from build123d import *

# Parameters (mm, degrees)
BOSS_EXTRUDE1_DEPTH     = 12.5
SKETCH2_W               = 12.5
SKETCH2_H               = 1.5
BOSS_EXTRUDE2_DEPTH     = 6
SKETCH3_R               = 1.5
CUT_EXTRUDE1_DEPTH      = 34.000006013
CUT_EXTRUDE1_DEPTH_BACK = 13.999994598
SKETCH5_W               = 1
SKETCH5_H               = 5
CUT_EXTRUDE2_DEPTH      = 24.499994598


with BuildPart() as part:
    # Sketch1 → Boss-Extrude1 (new body)
    with BuildSketch(Plane.XY):
        with BuildLine():
            Line((5.5, 17), (5.5, -18))
            ThreePointArc((5.5, -18), (-2.701e-06, -23.499994598), (-5.5, -17.999994598))
            Line((-5.5, -17.999994598), (-5.5, 17.000006013))
            ThreePointArc((-5.5, 17.000006013), (3.006e-06, 22.500006013), (5.5, 17))
        make_face()
        with BuildLine():
            Line((2.5, 17.5), (2.5, -17.5))
            ThreePointArc((2.5, -17.5), (0, -20), (-2.5, -17.5))
            Line((-2.5, -17.5), (-2.5, 17.5))
            ThreePointArc((-2.5, 17.5), (0, 20), (2.5, 17.5))
        make_face(mode=Mode.SUBTRACT)
    extrude(amount=BOSS_EXTRUDE1_DEPTH)

    # Sketch2 → Boss-Extrude2 (add)
    with BuildSketch(Plane(origin=(5.5, 0, 0), x_dir=(0, 0, -1), z_dir=(1, 0, 0))):
        with Locations((-6.25, -11.25)):
            Rectangle(SKETCH2_W, SKETCH2_H)
        with Locations((-6.25, -6.75)):
            Rectangle(SKETCH2_W, SKETCH2_H)
    extrude(amount=BOSS_EXTRUDE2_DEPTH)

    # Sketch3 → Cut-Extrude1 (cut, two sides)
    with BuildSketch(Plane(origin=(0, -10.5, 0), x_dir=(1, 0, 0), z_dir=(0, 1, 0))) as cut_extrude1_sk:
        with Locations((8.5, -3)):
            Circle(SKETCH3_R)
        with Locations((8.5, -9.5)):
            Circle(SKETCH3_R)
    extrude(amount=CUT_EXTRUDE1_DEPTH, mode=Mode.SUBTRACT)
    extrude(cut_extrude1_sk.sketch, amount=-CUT_EXTRUDE1_DEPTH_BACK, mode=Mode.SUBTRACT)

    # Sketch5 → Cut-Extrude2 (cut, through all)
    with BuildSketch(Plane(origin=(0, 0, 0), x_dir=(1, 0, 0), z_dir=(0, 1, 0))):
        with Locations((0, -6.25)):
            Rectangle(SKETCH5_W, SKETCH5_H)
    extrude(amount=-CUT_EXTRUDE2_DEPTH, mode=Mode.SUBTRACT)


solid = part.part
Here's how the part is built. I have some questions about the finished solid (model axes, mm). A direction names the side the tool comes from. Round coordinates to 2 decimals unless told otherwise and drop trailing zeros. Order: outer loops, then holes, each group sorted by start corner. A loop starts at its lowest first (then second) coordinate and runs counter-clockwise, first axis right, second up. Notation, with made-up numbers: M -24.75,-17.5 L -11.75,-17.5 A18 ccw -11.75,-8.5 Z; hole C 38,-19.5 d2. An arc over 180 degrees is marked long. Return JSON: item names as keys, results as strings. Group by question number.
1. If we section it at B-B on y = 2.5: List the corners of the cut face in (x, z) for me.
2. I'm going to push flat-ended pins straight in: pin 1 Ø5 at (y, z) = (-16, 8.5) entering from +X; pin 2 Ø2 at (x, y) = (4, 12.5) entering from -Z; pin 3 Ø1.1 at (y, z) = (-21, 5) entering from +X; pin 4 Ø3 at (x, z) = (8.5, 5.5) entering from -Y. Where does each tip first touch, or does it pass through?
3. If we mould it in two halves opening along X, with no side actions, what happens to faces 1 (the face through (1.994, -23.126, 6.162)), 2 (the face through (0, -22, 3.75)), 3 (the face through (-3, 0, 0))? For each: pulls with the +X half, pulls with the -X half, needs draft (parallel to the pull), parting line crosses it, or undercut.
4. If we section it at A-A on z = 9.5: List the corners of the cut face in (x, y) for me.
5. Please list where these lines run through material, in increasing order: probe 1 along X at (y, z) = (-10.95, 9.5); probe 2 along Z at (x, y) = (8.5, -11.4); probe 3 along X at (y, z) = (2.5, 1.5).
6. If we section it at C-C on x = 0: List the corners of the cut face in (y, z) for me, then the cut area to 3 significant figures.
7. If we section it at D-D on x = 8.5: List the corners of the cut face in (y, z) for me.
8. On a 3-axis mill with a long thin cutter (end or side, diameter ignored), from which of +Z, -Z, +X, -X, +Y, -Y can I reach the whole of each face in a straight line? I mean faces 4 (the face through (-0.8, -19.87, 6.16)), 5 (the face through (8, -10.5, 6)), 6 (the face through (0.5, -22, 6)). Say none if no direction works.
Reply:
{
 "1": {"outline": "M -5.5,0 L -2.5,0 L -2.5,12.5 L -5.5,12.5 Z; M 2.5,0 L 5.5,0 L 5.5,12.5 L 2.5,12.5 Z"},
 "2": {"pin 1": "x = 5.5", "pin 2": "z = 0", "pin 3": "x = 4.92", "pin 4": "y = -12"},
 "3": {"face 1": "parting line crosses it", "face 2": "undercut", "face 3": "needs draft"},
 "4": {"outline": "M -5.5,-18 A5.5 ccw 5.5,-18 L 5.5,-12 L 7,-12 L 7,-10.5 L 5.5,-10.5 L 5.5,-7.5 L 7,-7.5 L 7,-6 L 5.5,-6 L 5.5,17 A5.5 ccw -5.5,17 Z; M 10,-12 L 11.5,-12 L 11.5,-10.5 L 10,-10.5 Z; M 10,-7.5 L 11.5,-7.5 L 11.5,-6 L 10,-6 Z; hole M -2.5,-17.5 A2.5 ccw 2.5,-17.5 L 2.5,17.5 A2.5 ccw -2.5,17.5 Z"},
 "5": {"probe 1": "-5.5 to -2.5, 2.5 to 7, 10 to 11.5", "probe 2": "0 to 1.5, 4.5 to 8, 11 to 12.5", "probe 3": "-5.5 to -2.5, 2.5 to 5.5"},
 "6": {"outline": "M -23.5,0 L -20,0 L -20,3.75 L -23.5,3.75 Z; M -23.5,8.75 L -20,8.75 L -20,12.5 L -23.5,12.5 Z; M 20,0 L 22.5,0 L 22.5,12.5 L 20,12.5 Z", "area": "57.5 mm^2"},
 "7": {"outline": "M -12,0 L -10.5,0 L -10.5,1.5 L -12,1.5 Z; M -12,4.5 L -10.5,4.5 L -10.5,8 L -12,8 Z; M -12,11 L -10.5,11 L -10.5,12.5 L -12,12.5 Z; M -7.5,0 L -6,0 L -6,1.5 L -7.5,1.5 Z; M -7.5,4.5 L -6,4.5 L -6,8 L -7.5,8 Z; M -7.5,11 L -6,11 L -6,12.5 L -7.5,12.5 Z"},
 "8": {"face 4": "+Z, -Z", "face 5": "+Z, -Z, +X", "face 6": "-Y"}
}
